The listing builds one solid part. Answer for the finished solid, in the listing's coordinates (mm). A direction names the side the tool comes from. Coordinates: 2 decimals unless noted, no trailing zeros. Write each loop counter-clockwise with the first axis right and the second up, starting at its lowest first coordinate (ties: lowest second). Pieces come first, ordered by that corner, then holes. Notation, with made-up numbers: M 35.5,18.5 L 53.5,18.5 A20 ccw 53.5,54.5 Z; hole C 81.25,-19 d1. An arc over 180 degrees is marked long. Answer as a JSON object with one key per item and string values. Group by question number.
Autodesk Inventor part; units mm, degrees
ref_plane "YZ Plane" through (0, 0, 0) normal (1, 0, 0) x (0, 1, 0)
ref_plane "XZ Plane" through (0, 0, 0) normal (0, 1, 0) x (-1, 0, 0)
ref_plane "XY Plane" through (0, 0, 0) normal (0, 0, 1) x (1, 0, 0)
sketch "Boceto1" plane through (0, 0, 0) normal (0, 0, 1) x (1, 0, 0)
  arc A0 (4.8153, 5.75) -> (5.0185, -5.5736) centre (0, 0) ccw
  line L0 (0, 12.1119) -> (0, -11.4197) construction
  line L1 (-11.1817, 0) -> (12.1806, 0) construction
  line L2 (4.9434, 0.75) -> (5.5, 0.75)
  line L3 (4.9434, -0.75) -> (5.5, -0.75)
  line L4 (5.5, -0.75) -> (5.5, 0.75)
  line L5 (-0.75, 4.9434) -> (-0.75, 5.5)
  line L6 (0.75, 5.5) -> (-0.75, 5.5)
  line L7 (0.75, 4.9434) -> (0.75, 5.5)
  line L8 (-4.9434, -0.75) -> (-5.5, -0.75)
  line L9 (-5.5, 0.75) -> (-5.5, -0.75)
  line L10 (-4.9434, 0.75) -> (-5.5, 0.75)
  line L11 (0.75, -4.9434) -> (0.75, -5.5)
  line L12 (-0.75, -5.5) -> (0.75, -5.5)
  line L13 (-0.75, -4.9434) -> (-0.75, -5.5)
  arc A1 (-0.75, 4.9434) -> (-4.9434, 0.75) centre (0, 0) ccw
  arc A2 (-4.9434, -0.75) -> (-0.75, -4.9434) centre (0, 0) ccw
  arc A3 (0.75, -4.9434) -> (4.9434, -0.75) centre (0, 0) ccw
  arc A4 (4.9434, 0.75) -> (0.75, 4.9434) centre (0, 0) ccw
  circle A5 centre (0, 0) radius 5 construction
  line L14 (-11.772, 7.5) -> (14.517, 7.5) construction
  line L15 (-11.772, -7.5) -> (14.517, -7.5) construction
  line L16 (4.8153, 5.75) -> (6.5, 5.75)
  line L17 (8.5, 7.75) -> (8.5, 21.6618)
  line L18 (14.1379, 25.75) -> (25.6337, 25.75)
  line L19 (11.5, 21.75) -> (11.5, 3.4624)
  arc A6 (6.5, 5.75) -> (8.5, 7.75) centre (6.5, 7.75) ccw
  line L20 (5.0185, -5.5736) -> (11.5, 0.2624)
  line L21 (11.5, 21.75) -> (27.5524, 21.75)
  line L22 (28.4921, 22.408) -> (30.4, 27.65)
  line L23 (30.4, 27.65) -> (32.4, 27.65)
  line L24 (32.9, 28.15) -> (32.9, 30.15)
  line L25 (32.4, 30.65) -> (28.1174, 30.65)
  line L26 (27.6475, 30.321) -> (26.1036, 26.079)
  line L27 (14.1379, 25.75) -> (14.1379, 25.75)
  line L28 (13.6379, 26.25) -> (10.488, 26.25)
  line L29 (10.0181, 25.921) -> (8.5302, 21.8328)
  line L30 (11.5, 0.2624) -> (11.5, 3.2624)
  line L31 (12.5556, 3.3624) -> (11.7894, 3.3624) construction
  line L32 (11.5, 3.4624) -> (11.4, 3.3624)
  line L33 (11.5, 3.2624) -> (11.4, 3.3624)
  arc A7 (32.4, 27.65) -> (32.9, 28.15) centre (32.4, 28.15) ccw
  arc A8 (32.9, 30.15) -> (32.4, 30.65) centre (32.4, 30.15) ccw
  arc A9 (28.1174, 30.65) -> (27.6475, 30.321) centre (28.1174, 30.15) ccw
  arc A10 (14.1379, 25.75) -> (13.6379, 26.25) centre (13.6379, 25.75) ccw
  arc A11 (10.488, 26.25) -> (10.0181, 25.921) centre (10.488, 25.75) ccw
  arc A12 (25.6337, 25.75) -> (26.1036, 26.079) centre (25.6337, 26.25) ccw
  arc A13 (27.5524, 21.75) -> (28.4921, 22.408) centre (27.5524, 22.75) ccw
  arc A14 (8.5302, 21.8328) -> (8.5, 21.6618) centre (9, 21.6618) ccw
  point P0 (25.9838, 25.75)
  point P1 (8.5, 21.75)
  point P2 (28.2526, 21.75)
  point P3 (32.9, 27.65)
  point P4 (32.9, 30.65)
  point P5 (27.7673, 30.65)
  point P6 (14.1379, 26.25)
  point P7 (10.1379, 26.25)
  dimension "d0" = 15
  dimension "d4" = 0.75
  dimension "d6" = 1.5
  dimension "d11" = 360
  dimension "d13" = 10
  dimension "d14" = 0.5
  dimension "d15" = 5
  dimension "d16" = 1.75
  dimension "d22" = 3
  dimension "d27" = 20
  dimension "d49" = 2
  dimension "d89" = 4
  dimension "d90" = 3
  dimension "d91" = 3.5
  dimension "d92" = 4
  dimension "d93" = 0.5
  dimension "d96" = 2.5
  dimension "d97" = 4.5
  dimension "d98" = 3
  dimension "d100" = 48
  dimension "d101" = 0.2
  dimension "d102" = 0.1
  dimension "d106" = 0.1
  dimension "d108" = 70
  dimension "d111" = 24.4
  dimension "d113" = 19
  dimension "d118" = 70
  dimension "d123" = 0.5
  dimension "d124" = 1
  dimension "d125" = 0.5
  dimension "d155" = 8.9
  dimension "d156" = 38.15
extrude "Extrusión1" add sketch "Boceto1" against normal blind 46
sketch "Boceto2" plane through (11.5, 21.75, 0) normal (0, -1, 0) x (1, 0, 0)
  line L0 (10.4674, 0.9421) -> (10.4674, -47.0057) construction
  line L1 (16.0524, 0) -> (16.0524, -46)
  line L2 (0, 0) -> (0, -46)
  line L3 (-0.8036, -23) -> (23.8698, -23) construction
  line L4 (0, 0) -> (16.0524, 0)
  line L5 (16.0524, -46) -> (0, -46)
  circle A0 centre (10.4674, -23) radius 2.5
  circle A1 centre (10.4674, -23) radius 4.5
  circle A2 centre (10.4674, -38) radius 2.5
  circle A3 centre (10.4674, -38) radius 4.5
  circle A4 centre (10.4674, -8) radius 2.5
  circle A5 centre (10.4674, -8) radius 4.5
  point P0 (-11.5, 0)
  dimension "d134" = 5.585
  dimension "d136" = 23
  dimension "d137" = 23
  dimension "d138" = 5
  dimension "d139" = 9
  dimension "d140" = 2
  dimension "d143" = 15
hole "Agujero2" at (21.9674, 21.75, -8) at (21.9674, 21.75, -23) at (21.9674, 21.75, -38) direction (0, 1, 0) diameter 5 end through all countersink diameter 9 countersink angle 90
properties part number "HIN-61 BISAGRA (P2)" material "Aluminio"
Item 1: A cutting plane is placed at D-D, the plane y = 27. Write down the section's boundary in (x, z), and give its area (3 significant figures).
Item 2: A cutting plane is placed at B-B, the plane z = -38. State how many separate pieces and enclosed holes the cut face has, and give its area (3 significant figures).
Item 3: A cutting plane is placed at A-A, the plane x = 2.5. Write down the section's boundary in (y, z).
Item 4: Flat-ended cylindrical pins translate along their axes: pin 1 Ø1 at (y, z) = (14, -15.5) entering from +X; pin 2 Ø3 at (x, z) = (5, -34) entering from +Y; pin 3 Ø15.5 at (y, z) = (13.5, -15.5) entering from -X. Find the tip coordinate at first contact, or state that the pin passes through.
Item 5: A tool of negligible diameter and unlimited length cuts with its end or side. For faces 1 (the face through (8.5, 15, -23)), 2 (the face through (11.5, 2, -23)), 3 (the face through (5.5, 0, -23)), 4 (the face through (24.181, 23.625, -24.411)), 5 (the face through (10, 12, 0)), from which of +Z, -Z, +X, -X, +Y, -Y can it reach the whole face along a straight path? Write none if from no direction.
Item 6: For a pull along Y with two mould halves and no side action, classify faces 6 (the face through (0, -5.5, -23)), 7 (the face through (23.742, 23.625, -6.065)), 8 (the face through (-7.5, 0.1, -22.7)), 9 (the face through (-3.57, -3.5, -22.68)) as +Y half, -Y half, draft (parallel to the pull), parting line (faces both ways), or undercut.
Item 7: A cutting plane is placed at C-C, the plane y = 8.5. Write down the section's boundary in (x, z).
Item 8: Consider L1, parallel to X at y = 24, z = -8; L2, parallel to Y at x = 15, z = -13.5; L3, parallel to X at y = -3, z = -15. Determine where each line is inside the solid, lowest interval first. Write a range as from..to.
Answer:
{
 "1": {"outline": "M 26.44,-46 L 30.16,-46 L 30.16,0 L 26.44,0 Z", "area": "171 mm2"},
 "2": {"separate pieces": "2", "enclosed holes": "1", "area": "260 mm2"},
 "3": {"outline": "M -7.07,-46 L -4.33,-46 L -4.33,0 L -7.07,0 Z; M 4.33,-46 L 7.07,-46 L 7.07,0 L 4.33,0 Z"},
 "4": {"pin 1": "x = 11.5", "pin 2": "y = 6.63", "pin 3": "x = -4.82"},
 "5": {"face 1": "+Z, -Z, -X, +Y", "face 2": "+Z, -Z, +X, -Y", "face 3": "+Z, -Z", "face 4": "-Y", "face 5": "+Z, +X, -X, +Y, -Y"},
 "6": {"face 6": "undercut", "face 7": "-Y half", "face 8": "parting line", "face 9": "undercut"},
 "7": {"outline": "M 8.5,-46 L 11.5,-46 L 11.5,0 L 8.5,0 Z"},
 "8": {"L1": "9.32..19.47, 24.47..29.07", "L2": "21.75..25.75", "L3": "-6.87..-4, 4..7.88"}
}
